Autodesk Inventor part; units mm, degrees
ref_plane "YZ Plane" through (0, 0, 0) normal (1, 0, 0) x (0, 1, 0)
ref_plane "XZ Plane" through (0, 0, 0) normal (0, 1, 0) x (-1, 0, 0)
ref_plane "XY Plane" through (0, 0, 0) normal (0, 0, 1) x (1, 0, 0)
sketch "Sketch1" plane through (0, 0, 0) normal (0, 0, 1) x (1, 0, 0)
  line L0 (-15.875, -31.75) -> (15.875, -31.75)
  line L1 (15.875, -31.75) -> (15.875, 31.75)
  line L2 (15.875, 31.75) -> (-15.875, 31.75)
  line L3 (-15.875, 31.75) -> (-15.875, -31.75)
  line L4 (-15.875, -31.75) -> (15.875, 31.75) construction
  line L5 (15.875, -31.75) -> (-15.875, 31.75) construction
  point P0 (0, 0)
  dimension "height" = 63.5
  dimension "width" = 31.75
extrude "Extrusion1" add sketch "Sketch1" against normal blind 12.7
sketch "Sketch3" plane through (0, 0, 0) normal (0, 0, 1) x (1, 0, 0)
  line L0 (-15.875, -9.525) -> (15.875, -9.525)
  line L1 (15.875, -9.525) -> (15.875, 9.525)
  line L2 (15.875, 9.525) -> (-15.875, 9.525)
  line L3 (-15.875, 9.525) -> (-15.875, -9.525)
  line L4 (-15.875, -9.525) -> (15.875, 9.525) construction
  line L5 (15.875, -9.525) -> (-15.875, 9.525) construction
  line L6 (15.875, 31.75) -> (-15.875, 31.75)
  point P0 (0, 0)
  dimension "Channel_Width" = 19.05
  dimension "d52" = 31.75
extrude "Extrusion3" add sketch "Sketch3" along normal blind 44.45
sketch "Sketch6" plane through (15.875, -31.75, -12.7) normal (1, 0, 0) x (0, 0, -1)
  line L0 (-12.7, 31.75) -> (-57.15, 31.75) construction
  line L1 (-57.15, 22.225) -> (-57.15, 41.275) construction
  line L2 (-12.7, 41.275) -> (-12.7, 63.5) construction
  point P0 (-44.45, 31.75)
  dimension "d53" = 31.75
hole "Hole5" at (15.875, 0, 31.75) direction (-1, 0, 0) diameter 9.7282 end through all
sketch "Sketch13" plane through (15.875, -31.75, -12.7) normal (1, 0, 0) x (0, 0, -1)
  line L0 (-12.7, 63.5) -> (0, 63.5)
  line L1 (0, 0) -> (-6.35, 0)
  line L2 (-6.35, 0) -> (-6.35, 63.5)
  line L3 (-6.35, 63.5) -> (0, 63.5)
  line L4 (0, 63.5) -> (0, 0)
  point P0 (-12.7, 31.75)
  dimension "d98" = 6.35
extrude "Extrusion5" cut sketch "Sketch13" against normal through all
sketch "Sketch14" plane through (-15.875, -31.75, 0) normal (-1, 0, 0) x (0, 0, 1)
  line L0 (0, 0) -> (-6.35, 0)
  line L1 (0, 0) -> (0, 22.225)
  line L2 (-6.35, 0) -> (0, 0)
  line L3 (0, 0) -> (0, 6.604)
  line L4 (0, 6.604) -> (-6.35, 6.604)
  line L5 (-6.35, 6.604) -> (-6.35, 0)
  point P0 (0, 31.75)
  dimension "d101" = 6.604
extrude "Extrusion6" cut sketch "Sketch14" against normal through all
sketch "Sketch15" plane through (-15.875, 9.525, 0) normal (0, 1, 0) x (1, 0, 0)
  line L0 (31.75, -44.45) -> (0, -44.45)
  line L1 (0, 0) -> (0, -44.45)
  point P0 (15.875, 0)
  point P1 (15.875, -19.05)
  dimension "d104" = 25.4
  dimension "d123" = 15.875
hole "Hole11" at (0, 9.525, 19.05) direction (0, -1, 0) diameter 4.9784 end through all
sketch "Sketch11" plane through (0, 0, 44.45) normal (0, 0, 1) x (1, 0, 0)
  point P0 (0, 0)
hole "Hole12" at (0, 0, 44.45) direction (0, 0, -1) diameter 4.9784 depth 12.7 tip angle 118
sketch "Sketch16" plane through (15.875, 9.525, 0) normal (1, 0, 0) x (0, 0, -1)
  point P0 (0, -9.525)
sketch "Sketch17" plane through (0, 0, 0) normal (0, 0, 1) x (1, 0, 0)
  line L0 (-15.875, 31.75) -> (-15.875, 9.525)
  line L1 (-15.875, 9.525) -> (15.875, 9.525)
  line L2 (-15.875, 31.75) -> (15.875, 31.75)
  line L3 (15.875, 31.75) -> (15.875, 9.525)
  line L4 (15.875, 9.525) -> (-15.875, 9.525)
  line L5 (-15.875, 9.525) -> (-15.875, 31.75)
  point P0 (0, 0)
extrude "Extrusion7" cut sketch "Sketch17" against normal blind 0.381
sketch "Sketch18" plane through (0, 0, 0) normal (0, 0, 1) x (1, 0, 0)
  line L0 (-15.875, -25.146) -> (15.875, -25.146)
  line L1 (15.875, -9.525) -> (15.875, 9.525)
  line L2 (-15.875, -25.146) -> (15.875, -25.146)
  line L3 (15.875, -25.146) -> (15.875, -9.525)
  line L4 (15.875, -9.525) -> (-15.875, -9.525)
  line L5 (-15.875, -9.525) -> (-15.875, -25.146)
  point P0 (0, 0)
extrude "Extrusion8" cut sketch "Sketch18" against normal blind 0.381
sketch "Sketch10" plane through (0, 0, 44.45) normal (0, 0, 1) x (1, 0, 0)
  point P0 (0, 0)
sketch "Sketch12" plane through (-15.875, -9.525, 0) normal (0, -1, 0) x (1, 0, 0)
  point P0 (15.875, 15.875)
equation "\"d52\" = width"
properties part number "AsBuilt Support For Arms" material "Aluminum 6061"
Design review of the part built by this model. Coordinates are the model's own, in mm. A direction names the side the tool comes from. Coordinates: 2 decimals unless noted, no trailing zeros. Write each loop counter-clockwise with the first axis right and the second up, starting at its lowest first coordinate (ties: lowest second). Pieces come first, ordered by that corner, then holes. Notation, with made-up numbers: M 35.25,24 L 63.25,24 A27 ccw 63.25,53 Z; hole C 40.25,9.25 d11. An arc over 180 degrees is marked long. Answer as a JSON object with one key per item and string values.
Item 1: Draft analysis for pull direction X (two halves, no side actions). For faces 1 (the flat face through (15.875, 3, 14)), 2 (the cylindrical face through (-0.109, 2.487, 40.13)), 3 (the flat face through (0, 31.75, -3)), 4 (the cylindrical face through (-0.109, -0.133, 16.563)), state which applies: pulls with the +X half, pulls with the -X half, needs draft (parallel to the pull), parting line crosses it, or undercut.
Outcome:
{"face 1": "pulls with the +X half", "face 2": "undercut", "face 3": "needs draft", "face 4": "undercut"}
Item 2: Add section C-C, the plane x = 6. Give the boundary of the cut face in (y, z) (3 decimals).
Outcome:
{"outline": "M -25.146,-6.35 L 31.75,-6.35 L 31.75,-0.381 L 9.525,-0.381 L 9.525,44.45 L -9.525,44.45 L -9.525,-0.381 L -25.146,-0.381 Z; hole C 0,31.75 d9.728"}
Item 3: Insertion check: pin 1 Ø11 at (x, y) = (4.5, 20.5) entering from +Z; pin 2 Ø4 at (x, z) = (-3.5, 4) entering from +Y (3 decimals); pin 3 Ø4.5 at (x, y) = (0, 0) entering from +Z. Each pin has a flat end and moves straight along its axis. Give the tip position at first contact, or say it passes through.
Outcome:
{"pin 1": "z = -0.38", "pin 2": "y = 9.525", "pin 3": "z = 27.44"}
Item 4: Add section B-B, the plane y = 0. Give the boundary of the cut face in (x, z) (3 decimals), and give its area (3 significant figures).
Outcome:
{"outline": "M -15.875,-6.35 L 15.875,-6.35 L 15.875,26.886 L -15.875,26.886 Z; M -15.875,36.614 L -2.489,36.614 L -2.489,44.45 L -15.875,44.45 Z; M 2.489,36.614 L 15.875,36.614 L 15.875,44.45 L 2.489,44.45 Z; hole C 0,19.05 d4.978", "area": "1,250 mm²"}
Item 5: Add section D-D, the plane z = 31.75. Give the boundary of the cut face in (x, y) (3 decimals).
Outcome:
{"outline": "M -15.875,-9.525 L 15.875,-9.525 L 15.875,-4.864 L -15.875,-4.864 Z; M -15.875,4.864 L 15.875,4.864 L 15.875,9.525 L -15.875,9.525 Z"}
Item 6: Add section A-A, the plane z = 19.05. Give the boundary of the cut face in (x, y) (3 decimals).
Outcome:
{"outline": "M -15.875,-9.525 L -2.489,-9.525 L -2.489,9.525 L -15.875,9.525 Z; M 2.489,-9.525 L 15.875,-9.525 L 15.875,9.525 L 2.489,9.525 Z"}
Item 7: Machinability: for faces 5 (the flat face through (0, -9.525, 22)), 6 (the flat face through (0, 9.525, 22)), 7 (the flat face through (0, 3, -6.35)), which of the approach directions +Z, -Z, +X, -X, +Y, -Y give a long, thin tool a straight path to every point of the face, cutting with its end or side? Answer none if there is none.
Outcome:
{"face 5": "+Z, +X, -X, -Y", "face 6": "+Z, +X, -X, +Y", "face 7": "-Z, +X, -X, +Y, -Y"}
Item 8: Wall thickness on probe 1 along Y at (x, z) = (0, 40.25) (3 decimals); probe 2 along X at (y, z) = (2.75, 19.05) (3 decimals); probe 3 along Y at (x, z) = (3.5, 31.75) (3 decimals): over which ranges is each line inside the solid? List them lowest first.
Outcome:
{"probe 1": "-9.525 to -2.489, 2.489 to 9.525", "probe 2": "-15.875 to -2.489, 2.489 to 15.875", "probe 3": "-9.525 to -4.864, 4.864 to 9.525"}
